from build123d import *

# Parameters (mm, degrees)
SKETCH2_W           = 457.2
SKETCH2_H           = 609.6
BOSS_EXTRUDE1_DEPTH = 12.7
SKETCH3_R           = 14.3383
SKETCH3_R_2         = 2.38125
CUT_EXTRUDE1_DEPTH  = 382.211607903
FILLET1_R           = 6.35


with BuildPart() as part:
    # Sketch2 → Boss-Extrude1 (new body)
    with BuildSketch(Plane(origin=(0, 0, 0), x_dir=(1, 0, 0), z_dir=(0, 1, 0))):
        Rectangle(SKETCH2_W, SKETCH2_H)
    extrude(amount=BOSS_EXTRUDE1_DEPTH)

    # Sketch3 → Cut-Extrude1 (cut, through all)
    with BuildSketch(Plane(origin=(0, 12.7, 0), x_dir=(1, 0, 0), z_dir=(0, 1, 0))):
        with Locations(Location((-177.8, 203.2, 0), (0, 0, 270))):
            Circle(SKETCH3_R)
        with Locations(Location((-195.760512242, 221.160512242, 0), (0, 0, 270))):
            Circle(SKETCH3_R_2)
        with Locations(Location((-159.839487758, 221.160512242, 0), (0, 0, 270))):
            Circle(SKETCH3_R_2)
        with Locations(Location((-159.839487758, 185.239487758, 0), (0, 0, 270))):
            Circle(SKETCH3_R_2)
        with Locations(Location((-195.760512242, 185.239487758, 0), (0, 0, 270))):
            Circle(SKETCH3_R_2)
        with Locations(Location((195.760512242, 185.239487758, 0), (0, 0, 90))):
            Circle(SKETCH3_R_2)
        with Locations(Location((159.839487758, 185.239487758, 0), (0, 0, 90))):
            Circle(SKETCH3_R_2)
        with Locations(Location((159.839487758, 221.160512242, 0), (0, 0, 90))):
            Circle(SKETCH3_R_2)
        with Locations(Location((195.760512242, 221.160512242, 0), (0, 0, 90))):
            Circle(SKETCH3_R_2)
        with Locations(Location((177.8, 203.2, 0), (0, 0, 90))):
            Circle(SKETCH3_R)
        with Locations(Location((177.8, 139.7, 0), (0, 0, 270))):
            Circle(SKETCH3_R)
        with Locations(Location((195.760512242, 121.739487758, 0), (0, 0, 270))):
            Circle(SKETCH3_R_2)
        with Locations(Location((159.839487758, 121.739487758, 0), (0, 0, 270))):
            Circle(SKETCH3_R_2)
        with Locations(Location((159.839487758, 157.660512242, 0), (0, 0, 270))):
            Circle(SKETCH3_R_2)
        with Locations(Location((195.760512242, 157.660512242, 0), (0, 0, 270))):
            Circle(SKETCH3_R_2)
        with Locations(Location((-195.760512242, 157.660512242, 0), (0, 0, 90))):
            Circle(SKETCH3_R_2)
        with Locations(Location((-159.839487758, 157.660512242, 0), (0, 0, 90))):
            Circle(SKETCH3_R_2)
        with Locations(Location((-159.839487758, 121.739487758, 0), (0, 0, 90))):
            Circle(SKETCH3_R_2)
        with Locations(Location((-195.760512242, 121.739487758, 0), (0, 0, 90))):
            Circle(SKETCH3_R_2)
        with Locations(Location((-177.8, 139.7, 0), (0, 0, 90))):
            Circle(SKETCH3_R)
        with Locations(Location((177.8, 76.2, 0), (0, 0, 270))):
            Circle(SKETCH3_R)
        with Locations(Location((195.760512242, 58.239487758, 0), (0, 0, 270))):
            Circle(SKETCH3_R_2)
        with Locations(Location((159.839487758, 58.239487758, 0), (0, 0, 270))):
            Circle(SKETCH3_R_2)
        with Locations(Location((159.839487758, 94.160512242, 0), (0, 0, 270))):
            Circle(SKETCH3_R_2)
        with Locations(Location((195.760512242, 94.160512242, 0), (0, 0, 270))):
            Circle(SKETCH3_R_2)
        with Locations(Location((-195.760512242, 94.160512242, 0), (0, 0, 90))):
            Circle(SKETCH3_R_2)
        with Locations(Location((-159.839487758, 94.160512242, 0), (0, 0, 90))):
            Circle(SKETCH3_R_2)
        with Locations(Location((-159.839487758, 58.239487758, 0), (0, 0, 90))):
            Circle(SKETCH3_R_2)
        with Locations(Location((-195.760512242, 58.239487758, 0), (0, 0, 90))):
            Circle(SKETCH3_R_2)
        with Locations(Location((-177.8, 76.2, 0), (0, 0, 90))):
            Circle(SKETCH3_R)
        with Locations(Location((101.6, 76.2, 0), (0, 0, 270))):
            Circle(SKETCH3_R)
        with Locations(Location((119.560512242, 58.239487758, 0), (0, 0, 270))):
            Circle(SKETCH3_R_2)
        with Locations(Location((83.639487758, 58.239487758, 0), (0, 0, 270))):
            Circle(SKETCH3_R_2)
        with Locations(Location((83.639487758, 94.160512242, 0), (0, 0, 270))):
            Circle(SKETCH3_R_2)
        with Locations(Location((119.560512242, 94.160512242, 0), (0, 0, 270))):
            Circle(SKETCH3_R_2)
        with Locations(Location((101.6, 139.7, 0), (0, 0, 270))):
            Circle(SKETCH3_R)
        with Locations(Location((119.560512242, 121.739487758, 0), (0, 0, 270))):
            Circle(SKETCH3_R_2)
        with Locations(Location((83.639487758, 121.739487758, 0), (0, 0, 270))):
            Circle(SKETCH3_R_2)
        with Locations(Location((83.639487758, 157.660512242, 0), (0, 0, 270))):
            Circle(SKETCH3_R_2)
        with Locations(Location((119.560512242, 157.660512242, 0), (0, 0, 270))):
            Circle(SKETCH3_R_2)
        with Locations(Location((119.560512242, 185.239487758, 0), (0, 0, 90))):
            Circle(SKETCH3_R_2)
        with Locations(Location((83.639487758, 185.239487758, 0), (0, 0, 90))):
            Circle(SKETCH3_R_2)
        with Locations(Location((83.639487758, 221.160512242, 0), (0, 0, 90))):
            Circle(SKETCH3_R_2)
        with Locations(Location((119.560512242, 221.160512242, 0), (0, 0, 90))):
            Circle(SKETCH3_R_2)
        with Locations(Location((101.6, 203.2, 0), (0, 0, 90))):
            Circle(SKETCH3_R)
    extrude(amount=-CUT_EXTRUDE1_DEPTH, mode=Mode.SUBTRACT)

    # Fillet1
    fillet1_edges = [part.edges().sort_by_distance(p)[0] for p in [
        (228.6, 6.35, 304.8),
        (-228.6, 6.35, 304.8),
        (-228.6, 6.35, -304.8),
        (228.6, 6.35, -304.8),
    ]]
    fillet(fillet1_edges, radius=FILLET1_R)


solid = part.part
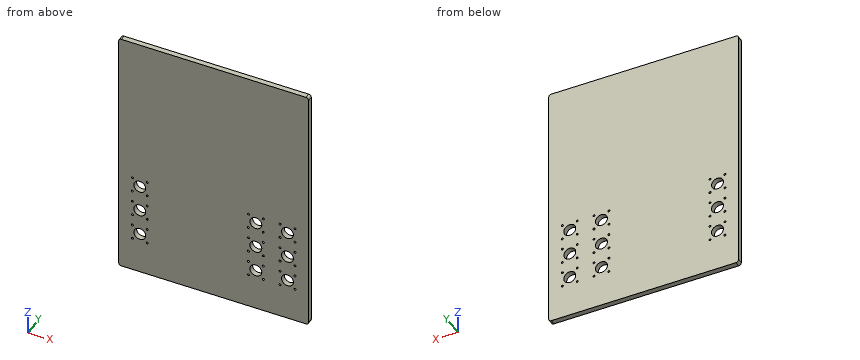
The listing builds one solid part. Answer for the finished solid, in the listing's coordinates (mm). Coordinates: 2 decimals unless noted, no trailing zeros. Loops run counter-clockwise (first coordinate to the right, second up) from the corner with the lowest first, then second, coordinate; pieces in that order, holes last. Notation, with made-up numbers: (30, 48.5) -> (50, 48.5) arc R22 ccw to (50, 81.5) -> close; hole circle Ø1 at (51, 3.5). An arc over 180 degrees is marked (long way). Answer in a Markdown table with one row per item. Add a question column.
1. The part is cut by section C-C, the plane y = 4. Count the separate pieces of the cut face and the enclosed holes in it, then the cut area to 3 significant figures.
2. The part is cut by section A-A, the plane z = -76.2. Write down the section's boundary in (x, y), then the cut area to 3 significant figures.
3. The part is cut by section B-B, the plane x = 177.8. Write down the section's boundary in (y, z), then the cut area to 3 significant figures.
4. A flat-ended cylindrical pin translates along its axis: P1, Ø4, axis at x = 83.64, z = -121.74, coming from the -Y side. Find the tip coordinate at first contact, or state that the pin passes through.
Answer below:
| question | item | result |
|---|---|---|
| 1 | separate pieces | 1 |
| 1 | enclosed holes | 45 |
| 1 | area | 272,000 mm2 |
| 2 | outline | (-228.6, 0) -> (-192.14, 0) -> (-192.14, 12.7) -> (-228.6, 12.7) -> close; (-163.46, 0) -> (87.26, 0) -> (87.26, 12.7) -> (-163.46, 12.7) -> close; (115.94, 0) -> (163.46, 0) -> (163.46, 12.7) -> (115.94, 12.7) -> close; (192.14, 0) -> (228.6, 0) -> (228.6, 12.7) -> (192.14, 12.7) -> close |
| 2 | area | 4,710 mm2 |
| 3 | outline | (0, -304.8) -> (12.7, -304.8) -> (12.7, -217.54) -> (0, -217.54) -> close; (0, -188.86) -> (12.7, -188.86) -> (12.7, -154.04) -> (0, -154.04) -> close; (0, -125.36) -> (12.7, -125.36) -> (12.7, -90.54) -> (0, -90.54) -> close; (0, -61.86) -> (12.7, -61.86) -> (12.7, 304.8) -> (0, 304.8) -> close |
| 3 | area | 6,650 mm2 |
| 4 | P1 | through |
